Read the model definition and answer for the solid it produces. Units are mm, in the model's axes. A direction names the side the tool comes from. Give positions to 0.01 mm unless a question says otherwise; leave off trailing zeros. Order: outer loops, then holes, each group sorted by start corner. A loop starts at its lowest first (then second) coordinate and runs counter-clockwise, first axis right, second up. Notation, with made-up numbers: (53, 57.25) - (68, 57.25) arc R21 cw to (68, 61.25) - close; hole circle Ø1 at (34.25, -38). An arc over 180 degrees is marked (long way). Write each question's results on one line, items separated by ' | '. Start each with the question number.
Q1. Find section A-A on x = 128. Give the vertices of the cut face in (y, z).
Q2. A tool of negligible diameter and unlimited length cuts with its end or side. For faces 1 (the face through (247.277, 13.198, 6.902)), 2 (the face through (205.5, 3, 7.1)), 3 (the face through (150.186, 21.386, 5.711)), from which of +Z, -Z, +X, -X, +Y, -Y can it reach the whole face along a straight path? Write none if from no direction.
Q3. Flat-ended cylindrical pins translate along their axes: P1, Ø3, axis at x = 152.5, y = 20, coming from the -Z side; P2, Ø0.8, axis at y = 0.5, z = 3.5, coming from the +X side; P3, Ø3.5, axis at x = 203, z = 7.5, coming from the -Y side. Find the tip coordinate at first contact, or state that the pin passes through.
Q4. For a pull along Y with two mould halves and no side action, classify faces 4 (the face through (306, 9, 7)), 5 (the face through (149.52, 21.6, 0.64)), 6 (the face through (53, 3, 7)), 7 (the face through (59, 15, 7)) as +Y half, -Y half, draft (parallel to the pull), parting line (faces both ways), or undercut.
Q5. Find the intervals of material crossed by line 1 along Y through (x, z) = (253, 8.25); line 2 along Y through (x, z) = (203, 6.75); line 3 along X through (y, z) = (18.25, 13), in increasing order. Write a range as from..to.
Q6. Find section B-B on x = 81.5. Give the vertices of the cut face in (y, z), and give its area (3 significant figures).
from build123d import *

# Parameters (mm, degrees)
ESQUISSE1_W                  = 306
ESQUISSE1_H                  = 26
BOSS_EXTRU_1_DEPTH           = 14
ENL_V_MAT_EXTRU_1_DEPTH      = 14.1
CONG_1_R                     = 1.5
CONG_2_R                     = 2
ENL_V_MAT_EXTRU_2_DEPTH      = 308.421534704
ENL_V_MAT_EXTRU_2_DEPTH_BACK = 308.421534704
CONG_3_R                     = 6
CONG_4_R                     = 4
ENL_V_MAT_EXTRU_3_DEPTH      = 308.421534704
ENL_V_MAT_EXTRU_3_DEPTH_BACK = 10
ESQUISSE4_R                  = 2.95
ESQUISSE6_R                  = 2.15
ENL_V_MAT_EXTRU_5_DEPTH      = 5.5
ENL_V_MAT_EXTRU_6_DEPTH      = 308.421534704
ENL_V_MAT_EXTRU_6_DEPTH_BACK = 308.421534704
ESQUISSE7_R                  = 6
ESQUISSE8_R                  = 3.65
ENL_V_MAT_EXTRU_7_DEPTH      = 1.3


with BuildPart() as part:
    # Esquisse1 → Boss.-Extru.1 (new body)
    with BuildSketch(Plane.XY):
        with Locations((153, 13)):
            Rectangle(ESQUISSE1_W, ESQUISSE1_H)
    extrude(amount=BOSS_EXTRU_1_DEPTH)

    # Esquisse2 → Enlèv. mat.-Extru.1 (cut)
    with BuildSketch(Plane.XY.offset(14)):
        with BuildLine():
            Line((215.053571921, 3), (190.946428079, 3))
            ThreePointArc((190.946428079, 3), (178, 18.1), (165.053571921, 3))
            Line((165.053571921, 3), (140.946428079, 3))
            ThreePointArc((140.946428079, 3), (128, 18.1), (115.053571921, 3))
            Line((115.053571921, 3), (90.946428079, 3))
            ThreePointArc((90.946428079, 3), (78, 18.1), (65.053571921, 3))
            Line((65.053571921, 3), (40.946428079, 3))
            ThreePointArc((40.946428079, 3), (28, 18.1), (15.053571921, 3))
            Line((15.053571921, 3), (3.9, 3))
            Line((3.9, 3), (3.9, 0))
            Line((3.9, 0), (302.1, 0))
            Line((302.1, 0), (302.1, 3))
            Line((302.1, 3), (290.946428079, 3))
            ThreePointArc((290.946428079, 3), (278, 18.1), (265.053571921, 3))
            Line((265.053571921, 3), (240.946428079, 3))
            ThreePointArc((240.946428079, 3), (228, 18.1), (215.053571921, 3))
        make_face()
    extrude(amount=-ENL_V_MAT_EXTRU_1_DEPTH, mode=Mode.SUBTRACT)

    # Congé1
    cong_1_edges = [part.edges().sort_by_distance(p)[0] for p in [
        (165.053571921, 3, 7),
        (190.946428079, 3, 7),
        (215.053571921, 3, 7),
        (240.946428079, 3, 7),
        (265.053571921, 3, 7),
        (290.946428079, 3, 7),
        (15.053571921, 3, 7),
        (40.946428079, 3, 7),
        (65.053571921, 3, 7),
        (90.946428079, 3, 7),
        (115.053571921, 3, 7),
        (140.946428079, 3, 7),
    ]]
    fillet(cong_1_edges, radius=CONG_1_R)

    # Congé2
    cong_2_edges = [part.edges().sort_by_distance(p)[0] for p in [
        (302.1, 3, 7),
        (3.9, 3, 7),
    ]]
    fillet(cong_2_edges, radius=CONG_2_R)

    # Esquisse3 → Enlèv. mat.-Extru.2 (cut, two sides: drawn at the far end of the back side and taken through both)
    with BuildSketch(Plane.XY.offset(14).offset(-ENL_V_MAT_EXTRU_2_DEPTH_BACK)):
        Polygon((0, 19), (50, 26), (0, 26), align=None)
        Polygon((306, 26), (306, 19), (256, 26), align=None)
    extrude(amount=ENL_V_MAT_EXTRU_2_DEPTH + ENL_V_MAT_EXTRU_2_DEPTH_BACK, mode=Mode.SUBTRACT)

    # Congé3
    cong_3_edges = [part.edges().sort_by_distance(p)[0] for p in [
        (0, 19, 7),
        (306, 19, 7),
    ]]
    fillet(cong_3_edges, radius=CONG_3_R)

    # Congé4
    # the kernel refuses this fillet: 4 mm, written as the material it takes off along each edge
    with BuildSketch(Plane(origin=(306, 0, -9.996874512), x_dir=(0, 1, 0), z_dir=(0, 0, 1))) as cong_4_piece_1:
        with BuildLine():
            CenterArc((3.998749805, 4), CONG_4_R, 181.432543738, 88.567456262)
            Line((0, 3.9), (-0.079974996, 3.898))
            ThreePointArc((-0.079974996, 3.898), (-0.08, 1.95), (-0.08, 0))
            Line((-0.08, 0), (0, -0.08))
            Line((0, -0.08), (3.998749805, -0.08))
            Line((3.998749805, -0.08), (3.998749805, 0))
        make_face()
    extrude(amount=33.993749023, mode=Mode.SUBTRACT)
    with BuildSketch(Plane(origin=(0, 0, -9.996874512), x_dir=(0, 1, 0), z_dir=(0, 0, 1))) as cong_4_piece_2:
        with BuildLine():
            CenterArc((3.998749805, -4), CONG_4_R, 90, 88.567456262)
            Line((0, -3.9), (-0.079974996, -3.898))
            ThreePointArc((-0.079974996, -3.898), (-0.08, -1.95), (-0.08, 0))
            Line((-0.08, 0), (0, 0.08))
            Line((0, 0.08), (3.998749805, 0.08))
            Line((3.998749805, 0.08), (3.998749805, 0))
        make_face()
    extrude(amount=33.993749023, mode=Mode.SUBTRACT)

    # Esquisse4 → Enlèv. mat.-Extru.3 (cut, two sides: drawn at the far end of the back side and taken through both)
    with BuildSketch(Plane(origin=(0, 0, 0), x_dir=(-1, 0, 0), z_dir=(0, 0, -1)).offset(-ENL_V_MAT_EXTRU_3_DEPTH_BACK)):
        with Locations((-153, 20.5)):
            Circle(ESQUISSE4_R)
        with Locations(Location((-153, 8.5, 0), (0, 0, 180))):
            Circle(ESQUISSE4_R)
    extrude(amount=ENL_V_MAT_EXTRU_3_DEPTH + ENL_V_MAT_EXTRU_3_DEPTH_BACK, mode=Mode.SUBTRACT)

    # Esquisse6 → Enlèv. mat.-Extru.5 (cut)
    with BuildSketch(Plane.XZ.offset(-3)):
        with Locations(Location((298, 7, 0), (0, 0, 270))):
            Circle(ESQUISSE6_R)
        with Locations(Location((8, 7, 0), (0, 0, 192.380798917))):
            Circle(ESQUISSE6_R)
        with Locations(Location((103, 7, 0), (0, 0, 270))):
            Circle(ESQUISSE6_R)
        with Locations(Location((203, 7, 0), (0, 0, 90))):
            Circle(ESQUISSE6_R)
    extrude(amount=-ENL_V_MAT_EXTRU_5_DEPTH, mode=Mode.SUBTRACT)

    # Esquisse7 → Enlèv. mat.-Extru.6 (cut, two sides: drawn at the far end of the back side and taken through both)
    with BuildSketch(Plane.XY.offset(14).offset(-ENL_V_MAT_EXTRU_6_DEPTH_BACK)):
        with Locations(Location((53, 15, 0), (0, 0, 180))):
            Circle(ESQUISSE7_R)
        with Locations(Location((103, 15, 0), (0, 0, 180))):
            Circle(ESQUISSE7_R)
        with Locations(Location((203, 15, 0), (0, 0, 180))):
            Circle(ESQUISSE7_R)
        with Locations(Location((253, 15, 0), (0, 0, 180))):
            Circle(ESQUISSE7_R)
    extrude(amount=ENL_V_MAT_EXTRU_6_DEPTH + ENL_V_MAT_EXTRU_6_DEPTH_BACK, mode=Mode.SUBTRACT)

    # Esquisse8 → Enlèv. mat.-Extru.7 (cut)
    with BuildSketch(Plane(origin=(0, 0, 0), x_dir=(-1, 0, 0), z_dir=(0, 0, -1))):
        with Locations((-153, 20.5)):
            Circle(ESQUISSE8_R)
        with Locations((-153, 8.5)):
            Circle(ESQUISSE8_R)
    extrude(amount=-ENL_V_MAT_EXTRU_7_DEPTH, mode=Mode.SUBTRACT)


solid = part.part
Working result:
1) outline: (18.1, 0) - (26, 0) - (26, 14) - (18.1, 14) - close
2) face 1: +Z, -Z | face 2: +Z, -Z, -Y | face 3: -Z
3) P1: z = 10 | P2: x = 304.53 | P3: y = 3
4) face 4: draft | face 5: undercut | face 6: -Y half | face 7: undercut
5) line 1: 3..9, 21..26 | line 2: 8.5..9, 21..26 | line 3: 2..47.96, 58.04..97.96, 108.04..197.96, 208.04..247.96, 258.04..304
6) outline: (17.62, 0) - (26, 0) - (26, 14) - (17.62, 14) - close | area: 117 mm²
